```python
from build123d import *

# Parameters (mm, degrees)
F1_DEPTH = 3.175
F2_W     = 25.4
F2_H     = 12.7
F3_DEPTH = 3.175
F4_R     = 6.34999
F5_W     = 12.954
F5_H     = 3.175
F6_DEPTH = 25.4


# Not quite as in the source:
# - a fillet or chamfer is up to 0.001 mm smaller than in the source, because OpenCascade refuses the exact size


with BuildPart() as f1:
    # F0 (on Front) → F1 (new body)
    with BuildSketch(Plane.XZ):
        with BuildLine():
            ThreePointArc((0, 6.35), (1.8598719395, 1.8598719395), (6.35, 0))
            Line((6.35, 0), (38.1, 0))
            Line((38.1, 0), (38.1, 12.7))
            Line((38.1, 12.7), (6.35, 12.7))
            ThreePointArc((6.35, 12.7), (1.8598719395, 10.8401280605), (0, 6.35))
        make_face()
    extrude(amount=F1_DEPTH)

    # F2 (on face) → F3 (join)
    with BuildSketch(Plane.XZ.offset(3.175)):
        with Locations((25.4, 6.35)):
            Rectangle(F2_W, F2_H)
    extrude(amount=F3_DEPTH)

    # F4 (radius 6.35 in the source; OpenCascade refuses exactly that, so slightly less here)
    f4_edges = [f1.edges().sort_by_distance(p)[0] for p in [
        (38.1, -3.175, 12.7),
        (38.1, -3.175, 0),
    ]]
    fillet(f4_edges, radius=F4_R)

    # F5 (on face) → F6 (cut)
    with BuildSketch(Plane.XY.offset(12.7)):
        with Locations((31.75, -1.5875)):
            Rectangle(F5_W, F5_H)
    extrude(amount=-F6_DEPTH, mode=Mode.SUBTRACT)

    # F7: F1 across face


with BuildPart() as f1_1:
    add(f1.part)
    add(f1.part.mirror(Plane(origin=(13.2758554346, 0, 6.35), x_dir=(1, 0, 0), z_dir=(0, 1, 0))))


solid = f1_1.part
```
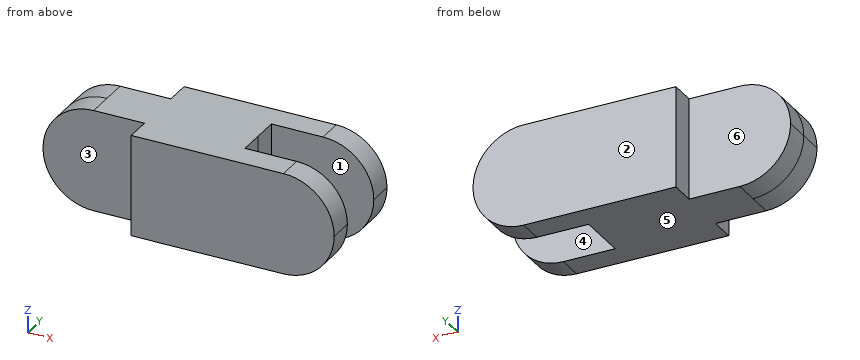
Geometry: final body of the model. Coordinates: model frame, mm. Face numbers are marked on the shaded views. A direction names the side the tool comes from. Coordinates: 2 decimals unless noted, no trailing zeros. Order: outer loops, then holes, each group sorted by start corner. A loop starts at its lowest first (then second) coordinate and runs counter-clockwise, first axis right, second up. Notation, with made-up numbers: (63.25, 83.5) - (84.25, 83.5) arc R33 ccw to (84.25, 114.5) - close; hole circle Ø8 at (-27, 31.25). An arc over 180 degrees is marked (long way). Return JSON: item names as keys, results as strings. Group by question number.
1. Cut plane A-A (x = 29.5). Output: boundary loops of the cut face in (y, z) (3 decimals), plus the area to 3 significant figures.
2. Pin query (flat end, axial travel): pin 1 (1 mm diameter, centred on y = 5, z = 3.5, fed in from -X); pin 2 (4 mm diameter, centred on x = 4.5, z = 7, fed in from -Y) (3 decimals); pin 3 (6.5 mm diameter, centred on x = 6, z = 8.5, fed in from +Y) (3 decimals). Return the tip coordinate at first contact, or that it passes through.
3. Cut plane B-B (z = 5.25). Output: boundary loops of the cut face in (x, y) (3 decimals).
4. Material intervals for line 1 along Y through (x, z) = (26, 6.5) (3 decimals); line 2 along Y through (x, z) = (8, 2) (3 decimals); line 3 along X through (y, z) = (-5, 9.75), sorted ascending. Write a range as [from, to].
5. Set-up query: the marked faces 1, 2 and 3. Return all of +Z, -Z, +X, -X, +Y, -Y with unobstructed straight access to the full face (end or side cutting, diameter ignored); none if empty.
6. Cut plane C-C (y = -2.5). Output: boundary loops of the cut face in (x, z), plus the area to 3 significant figures.
7. Cut plane D-D (x = 8.5). Output: boundary loops of the cut face in (y, z) (3 decimals).
8. Pull-direction query (Y, two-part tool) for the marked faces 4, 5 and 6; classes: pulls with the +Y half, pulls with the -Y half, needs draft (parallel to the pull), parting line crosses it, or undercut.
Resolved:
{
 "1": {"outline": "(-6.35, 0) - (-3.175, 0) - (-3.175, 12.7) - (-6.35, 12.7) - close; (3.175, 0) - (6.35, 0) - (6.35, 12.7) - (3.175, 12.7) - close", "area": "80.6 mm²"},
 "2": {"pin 1": "stops at x = 12.7", "pin 2": "stops at y = -3.175", "pin 3": "stops at y = 3.175"},
 "3": {"outline": "(0.096, -3.175) - (12.7, -3.175) - (12.7, -6.35) - (38.004, -6.35) - (38.004, -3.175) - (25.273, -3.175) - (25.273, 3.175) - (38.004, 3.175) - (38.004, 6.35) - (12.7, 6.35) - (12.7, 3.175) - (0.096, 3.175) - close"},
 "4": {"line 1": "y = [-6.35, -3.175], [3.175, 6.35]", "line 2": "y = [-3.175, 3.175]", "line 3": "x = [12.7, 37.11]"},
 "5": {"face 1": "+Z, -Z, +X", "face 2": "+Z, -Z, +X, -X, +Y", "face 3": "+Z, -Z, -X, -Y"},
 "6": {"outline": "(6.35, 0) - (25.27, 0) - (25.27, 12.7) - (6.35, 12.7) arc R6.35 ccw to start", "area": "304 mm²"},
 "7": {"outline": "(-3.175, 0) - (3.175, 0) - (3.175, 12.7) - (-3.175, 12.7) - close"},
 "8": {"face 4": "undercut", "face 5": "needs draft", "face 6": "pulls with the +Y half"}
}
